The model under review builds one solid part; all positions refer to its coordinate system, in mm. A direction names the side the tool comes from. Round coordinates to 2 decimals unless told otherwise and drop trailing zeros. Write each loop counter-clockwise with the first axis right and the second up, starting at its lowest first coordinate (ties: lowest second). Pieces come first, ordered by that corner, then holes.
Item 1: Add section B-B (x = 34). Give the boundary of the cut face in (y, z).
Item 2: Add section C-C (y = 19). Give the boundary of the cut face in (x, z).
Item 3: Machinability: for faces 1 (the face through (61.6, 82.2, -2)), 2 (the face through (8, 26, -4)), 3 (the face through (8, 82, -3)), 4 (the face through (-5, 52, -3)), 5 (the face through (27, 15.2, -1)), which of the approach directions +Z, -Z, +X, -X, +Y, -Y give a long, thin tool a straight path to every point of the face, cutting with its end or side? Answer none if there is none.
Item 4: Add section A-A (y = 10). Give the boundary of the cut face in (x, z).
Item 5: Clearance check with flat-ended pins moving along their axes: pin 1 Ø1.5 at (x, y) = (34, 49) entering from -Z; pin 2 Ø3 at (x, y) = (63, 48.5) entering from +Z; pin 3 Ø1 at (y, z) = (41, -3.5) entering from -X. State where each tip first meets the part, or that it passes through.
Item 6: Add section D-D (x = 54.5). Give the boundary of the cut face in (y, z).
Item 7: Draft analysis for pull direction Y (two halves, no side actions). For faces 6 (the face through (67.43, 0.6, -3.04)), 7 (the face through (11.18, 3.45, -3.75)), 8 (the face through (4, 46, -5)), state which applies: +Y half, -Y half, draft (parallel to the pull), parting line (faces both ways), or undercut.
Item 8: To check wall thickness, follow L1, parallel to X at y = 4.25, z = -3; L2, parallel to Y at x = 64, z = -2.9; L3, parallel to X at y = 27.5, z = -4.25. State the ranges of each line that lie inside material, in increasing order.
```python
from build123d import *

# Parameters (mm, degrees)
EXTRUDE_1_DEPTH          = 6
EXTRUDE_4_DEPTH          = 6.8
CUT_EXTRUDE_START        = -1.8
CUT_EXTRUDE_6_DEPTH      = 110.619208398
FILLET_1_R               = 2
CUT_EXTRUDE_4_DEPTH      = 112.419208398
CUT_EXTRUDE_4_DEPTH_BACK = 112.419208398
SKETCH_4_R               = 1.6
SKETCH_5_R               = 3.75
SKETCH_5_W               = 10.4
SKETCH_5_H               = 6.2
SKETCH_5_W_2             = 2.5
SKETCH_5_H_2             = 1
SKETCH_5_W_3             = 9.4
SKETCH_5_H_3             = 11.4
CUT_EXTRUDE_5_DEPTH      = 112.419208398
SKETCH_5_3_W             = 9.4
SKETCH_5_3_H             = 11.4
SKETCH_5_3_R             = 3.3
EXTRUDE_5_DEPTH          = 0.4
SKETCH_6_W               = 20
SKETCH_6_H               = 36
EXTRUDE_7_DEPTH          = 6
FILLET_2_R               = 2
FILLET_3_R               = 4
SKETCH_7_R               = 1.4
CUT_EXTRUDE_7_DEPTH      = 20
SKETCH_4_3_R             = 3
SKETCH_4_3_R_2           = 1.6
CUT_EXTRUDE_8_DEPTH      = 4
SKETCH_8_R               = 1.4
CUT_EXTRUDE_9_DEPTH      = 7
CHAMFER_1_SIZE           = 1.4


with BuildPart() as part:
    # 草图1 → 凸台-拉伸1 (new body)
    with BuildSketch(Plane.XY):
        Polygon((0, 0), (68, 0), (68, 88), (8, 88), (8, 52), (0, 52), align=None)
    extrude(amount=-EXTRUDE_1_DEPTH)

    # 草图1<2> → 凸台-拉伸4 (add)
    with BuildSketch(Plane.XY):
        Polygon((2.2, 49.8), (2.2, 2.2), (65.8, 2.2), (65.8, 85.8), (10.2, 85.8), (10.2, 49.8), align=None)
        Polygon((8, 44), (8, 8), (60, 8), (60, 80), (16, 80), (16, 44), align=None, mode=Mode.SUBTRACT)
    extrude(amount=-EXTRUDE_4_DEPTH)

    # 草图1<5> → 切除-拉伸6 (cut, through all)
    with BuildSketch(Plane.XY.offset(CUT_EXTRUDE_START)):
        Polygon((16, 80), (16, 44), (8, 44), (8, 8), (60, 8), (60, 80), align=None)
    extrude(amount=-CUT_EXTRUDE_6_DEPTH, mode=Mode.SUBTRACT)

    # 圆角1
    fillet_1_edges = [part.edges().sort_by_distance(p)[0] for p in [
        (68, 88, -3),
        (68, 0, -3),
        (0, 0, -3),
        (10.2, 85.8, -6.4),
        (65.8, 85.8, -6.4),
        (65.8, 2.2, -6.4),
        (2.2, 2.2, -6.4),
        (2.2, 49.8, -6.4),
    ]]
    fillet(fillet_1_edges, radius=FILLET_1_R)

    # 草图4 → 切除-拉伸4 (cut, two sides: drawn at the far end of the back side and taken through both)
    with BuildSketch(Plane.XY.offset(-CUT_EXTRUDE_4_DEPTH_BACK)):
        with Locations((12, 84)):
            Circle(SKETCH_4_R)
        with Locations((64, 84)):
            Circle(SKETCH_4_R)
        with Locations((64, 4)):
            Circle(SKETCH_4_R)
        with Locations((4, 48)):
            Circle(SKETCH_4_R)
        with Locations((4, 4)):
            Circle(SKETCH_4_R)
        with Locations((64, 48)):
            Circle(SKETCH_4_R)
    extrude(amount=CUT_EXTRUDE_4_DEPTH + CUT_EXTRUDE_4_DEPTH_BACK, mode=Mode.SUBTRACT)

    # 草图5 → 切除-拉伸5 (cut, through all)
    with BuildSketch(Plane.XY):
        with Locations((26.95, 20.7)):
            Circle(SKETCH_5_R)
        with Locations((42.8, 8.3)):
            Rectangle(SKETCH_5_W, SKETCH_5_H)
        with Locations((26.95, 14.7)):
            Rectangle(SKETCH_5_W_2, SKETCH_5_H_2)
        with Locations((53.3, 18.1)):
            Rectangle(SKETCH_5_W_3, SKETCH_5_H_3)
        with BuildLine():
            Line((39.8, 16.7), (45.8, 16.7))
            ThreePointArc((45.8, 16.7), (47.6, 18.5), (45.8, 20.3))
            Line((45.8, 20.3), (39.8, 20.3))
            ThreePointArc((39.8, 20.3), (38, 18.5), (39.8, 16.7))
        make_face()
    extrude(amount=-CUT_EXTRUDE_5_DEPTH, mode=Mode.SUBTRACT)

    # 草图5<3> → 凸台-拉伸5 (add)
    with BuildSketch(Plane.XY):
        with Locations((53.3, 18.1)):
            Rectangle(SKETCH_5_3_W, SKETCH_5_3_H)
        with Locations((53.3, 19)):
            Circle(SKETCH_5_3_R, mode=Mode.SUBTRACT)
    extrude(amount=-EXTRUDE_5_DEPTH)

    # 草图6 → 凸台-拉伸7 (add)
    with BuildSketch(Plane.XY):
        with Locations((-2, 70)):
            Rectangle(SKETCH_6_W, SKETCH_6_H)
    extrude(amount=-EXTRUDE_7_DEPTH)

    # 圆角2
    fillet_2_edges = [part.edges().sort_by_distance(p)[0] for p in [
        (0, 52, -3),
    ]]
    fillet(fillet_2_edges, radius=FILLET_2_R)

    # 圆角3
    fillet_3_edges = [part.edges().sort_by_distance(p)[0] for p in [
        (-12, 52, -3),
    ]]
    fillet(fillet_3_edges, radius=FILLET_3_R)

    # 草图7 → 切除-拉伸7 (cut)
    with BuildSketch(Plane.ZY.offset(12)):
        with Locations((-3, 82)):
            Circle(SKETCH_7_R)
        with Locations((-3, 62)):
            Circle(SKETCH_7_R)
    extrude(amount=-CUT_EXTRUDE_7_DEPTH, mode=Mode.SUBTRACT)

    # 草图4<3> → 切除-拉伸8 (cut)
    # profile 1 of 6: a face of its own
    with BuildSketch(Plane.XY):
        with Locations((12, 84)):
            Circle(SKETCH_4_3_R)
        with Locations((12, 84)):
            Circle(SKETCH_4_3_R_2, mode=Mode.SUBTRACT)
    # profile 2 of 6: a face of its own
    with BuildSketch(Plane.XY):
        with Locations((64, 84)):
            Circle(SKETCH_4_3_R)
        with Locations((64, 84)):
            Circle(SKETCH_4_3_R_2, mode=Mode.SUBTRACT)
    # profile 3 of 6: a face of its own
    with BuildSketch(Plane.XY):
        with Locations((4, 48)):
            Circle(SKETCH_4_3_R)
        with Locations((4, 48)):
            Circle(SKETCH_4_3_R_2, mode=Mode.SUBTRACT)
    # profile 4 of 6: a face of its own
    with BuildSketch(Plane.XY):
        with Locations((64, 48)):
            Circle(SKETCH_4_3_R)
        with Locations((64, 48)):
            Circle(SKETCH_4_3_R_2, mode=Mode.SUBTRACT)
    # profile 5 of 6: a face of its own
    with BuildSketch(Plane.XY):
        with Locations((4, 4)):
            Circle(SKETCH_4_3_R)
        with Locations((4, 4)):
            Circle(SKETCH_4_3_R_2, mode=Mode.SUBTRACT)
    # profile 6 of 6: a face of its own
    with BuildSketch(Plane.XY):
        with Locations((64, 4)):
            Circle(SKETCH_4_3_R)
        with Locations((64, 4)):
            Circle(SKETCH_4_3_R_2, mode=Mode.SUBTRACT)
    extrude(amount=-CUT_EXTRUDE_8_DEPTH, mode=Mode.SUBTRACT)

    # 草图8 → 切除-拉伸9 (cut)
    with BuildSketch(Plane.XZ):
        with Locations(Location((58, -3, 0), (0, 0, 270))):
            Circle(SKETCH_8_R)
        with Locations(Location((10, -3, 0), (0, 0, 270))):
            Circle(SKETCH_8_R)
        with Locations(Location((34, -3, 0), (0, 0, 270))):
            Circle(SKETCH_8_R)
    extrude(amount=-CUT_EXTRUDE_9_DEPTH, mode=Mode.SUBTRACT)

    # 倒角1
    chamfer_1_edges = [part.edges().sort_by_distance(p)[0] for p in [
        (2.4, 4, -4),
        (62.4, 48, -4),
        (2.4, 48, -4),
        (62.4, 84, -4),
        (62.4, 4, -4),
        (9, 84, -4),
    ]]
    chamfer(chamfer_1_edges, length=CHAMFER_1_SIZE - 0.0001)  # a hair under: the kernel refuses the full size


solid = part.part
```
Numbers:
1. outline: (0, -6) - (2.2, -6) - (2.2, -6.8) - (8, -6.8) - (8, -1.8) - (80, -1.8) - (80, -6.8) - (85.8, -6.8) - (85.8, -6) - (88, -6) - (88, 0) - (0, 0) - (0, -1.6) - (7, -1.6) - (7, -4.4) - (0, -4.4) - close
2. outline: (0, -6) - (2.2, -6) - (2.2, -6.8) - (8, -6.8) - (8, -1.8) - (23.61, -1.8) - (23.61, 0) - (0, 0) - close; (30.29, -1.8) - (38.07, -1.8) - (38.07, 0) - (30.29, 0) - close; (47.53, -1.8) - (48.6, -1.8) - (48.6, -0.4) - (50, -0.4) - (50, 0) - (47.53, 0) - close; (56.6, -0.4) - (58, -0.4) - (58, -1.8) - (60, -1.8) - (60, -6.8) - (65.8, -6.8) - (65.8, -6) - (68, -6) - (68, 0) - (56.6, 0) - close
3. face 1: +Z
3. face 2: -Z
3. face 3: -X
3. face 4: +Z, -Z, -X, -Y
3. face 5: +Z, -Z
4. outline: (0, -6) - (2.2, -6) - (2.2, -6.8) - (8, -6.8) - (8, -1.8) - (37.6, -1.8) - (37.6, 0) - (0, 0) - close; (48, -1.8) - (60, -1.8) - (60, -6.8) - (65.8, -6.8) - (65.8, -6) - (68, -6) - (68, 0) - (48, 0) - close
5. pin 1: stops at z = -1.8
5. pin 2: stops at z = -4.38
5. pin 3: stops at x = 0
6. outline: (0, -6) - (2.2, -6) - (2.2, -6.8) - (8, -6.8) - (8, -1.8) - (12.4, -1.8) - (12.4, -0.4) - (15.93, -0.4) - (15.93, 0) - (0, 0) - close; (22.07, -0.4) - (23.8, -0.4) - (23.8, -1.8) - (80, -1.8) - (80, -6.8) - (85.8, -6.8) - (85.8, -6) - (88, -6) - (88, 0) - (22.07, 0) - close
7. face 6: -Y half
7. face 7: draft
7. face 8: undercut
8. L1: x = 0 to 1.01, 6.99 to 8.6, 11.4 to 32.6, 35.4 to 56.6, 59.4 to 61.01, 66.99 to 68
8. L2: y = 0 to 1, 7 to 45, 51 to 81, 87 to 88
8. L3: x = 0 to 8, 60 to 68
